```python
from build123d import *

# Parameters (mm, degrees)
SKETCH1_R           = 11.5
SKETCH1_R_2         = 1.4999999999999991
SKETCH1_R_3         = 1.4999999999999987
SKETCH1_R_4         = 1.5000000000000009
SKETCH1_R_5         = 1.5000000000000002
BOSS_EXTRUDE1_DEPTH = 3.5
BOSS_EXTRUDE2_DEPTH = 17.5
CUT_EXTRUDE1_DEPTH  = 73.64483808227534
SKETCH4_R           = 1.3750000000000042
SKETCH4_R_2         = 1.375000000000001
CUT_EXTRUDE2_DEPTH  = 266.22147666332955
FILLET1_R           = 2.5
FILLET2_R           = 1


with BuildPart() as part:
    # Sketch1 → Boss-Extrude1 (new body)
    with BuildSketch(Plane.XY):
        with BuildLine():
            Line((-20.5, -16.000000000000007), (-15.999999999999996, -20.500000000000007))
            Line((-15.999999999999996, -20.500000000000007), (16.000000000000004, -20.5))
            Line((16.000000000000004, -20.5), (20.5, -16))
            Line((20.5, -16), (20.5, 16))
            Line((20.5, 16), (16.000000000000004, 20.5))
            Line((16.000000000000004, 20.5), (-23.500000000000007, 20.5))
            Line((-23.500000000000007, 20.5), (-23.500000000000007, 33))
            Line((-23.500000000000007, 33), (-41.00000000000001, 33))
            Line((-41.00000000000001, 33), (-41.00000000000001, 22.75))
            Line((-41.00000000000001, 22.75), (-35.22649730810378, 12.75))
            Line((-35.22649730810378, 12.75), (-29.500000000000007, 12.750000000000002))
            ThreePointArc((-29.500000000000007, 12.750000000000002), (-23.136038969321078, 10.11396103067893), (-20.500000000000004, 3.750000000000001))
            Line((-20.500000000000004, 3.750000000000001), (-20.5, -16.000000000000007))
        make_face()
        Circle(SKETCH1_R, mode=Mode.SUBTRACT)
        with Locations((-15.500000000000002, 15.5)):
            Circle(SKETCH1_R_2, mode=Mode.SUBTRACT)
        with Locations((15.500000000000002, 15.499999999999998)):
            Circle(SKETCH1_R_3, mode=Mode.SUBTRACT)
        with Locations((15.5, -15.5)):
            Circle(SKETCH1_R_4, mode=Mode.SUBTRACT)
        with Locations((-15.5, -15.5)):
            Circle(SKETCH1_R_5, mode=Mode.SUBTRACT)
        with Locations((-30.00000000000001, 20.746197723675813)):
            Circle(SKETCH1_R_4, mode=Mode.SUBTRACT)
    extrude(amount=BOSS_EXTRUDE1_DEPTH)

    # Sketch2 → Boss-Extrude2 (add)
    with BuildSketch(Plane.ZY.offset(41.00000000000001)):
        Polygon((3.5, 33), (20.15, 33), (20.15, 27.000000000000004), (3.5, 22.75), align=None)
    extrude(amount=-BOSS_EXTRUDE2_DEPTH)

    # Sketch3 → Cut-Extrude1 (cut, through all)
    with BuildSketch(Plane.ZY.offset(41.00000000000001)):
        with BuildLine():
            Line((0, 26.060862236758553), (0, 38.04576260464925))
            Line((0, 38.04576260464925), (20.15, 38.04576260464925))
            Line((20.15, 38.04576260464925), (20.149999999999995, 30.990381056766584))
            ThreePointArc((20.149999999999995, 30.990381056766584), (9.085499481104915, 32.57032381420525), (0, 26.060862236758553))
        make_face()
    extrude(amount=-CUT_EXTRUDE1_DEPTH, mode=Mode.SUBTRACT)

    # Sketch4 → Cut-Extrude2 (cut, through all)
    with BuildSketch(Plane(origin=(-1.4737e-13, -20.499999999999993, -236.3635116976825), x_dir=(1, 2.2e-16, 0), z_dir=(-2.2e-16, 1, 0))):
        with Locations((-35.99999999999985, -249.01351169768247)):
            Circle(SKETCH4_R)
        with Locations((-28.499999999999844, -249.01351169768247)):
            Circle(SKETCH4_R_2)
    extrude(amount=CUT_EXTRUDE2_DEPTH, mode=Mode.SUBTRACT)

    # Fillet1
    # the kernel refuses this fillet: 2.5 mm, written as the material it adds along each edge
    with BuildSketch(Plane(origin=(-41.00000000000001, 22.75, 3.5), x_dir=(0, -1, 0), z_dir=(1, 0, 0))) as fillet1_piece_1_section:
        with BuildLine():
            CenterArc((FILLET1_R * 0.776808330642, -FILLET1_R), FILLET1_R, 90, 75.68071687498136)
            Line((-FILLET1_R * 0.192124217376, -FILLET1_R * 0.752674875131), (0, 0))
            Line((0, 0), (FILLET1_R * 0.776808330642, 0))
        make_face()
    fillet1_piece_1 = extrude(amount=17.5, mode=Mode.PRIVATE)
    fillet1_piece_1 = split(fillet1_piece_1, bisect_by=Plane(origin=(-38.678687412646255, 18.729368658454117, 3.931557915234251), z_dir=(0.8660254037844398, 0.49999999999999795, 0)), keep=Keep.TOP, mode=Mode.PRIVATE)
    fillet1_piece_1 = fillet1_piece_1 - Plane(origin=(-30.00000000000001, 20.746197723675813, 3.931557915234251), x_dir=(1, 0, 0), z_dir=(0, 0, -1)) * Cylinder(1.5000000000000009, 43, mode=Mode.PRIVATE)
    add(fillet1_piece_1)
    # the kernel refuses this fillet: 2.5 mm, written as the material it takes off along each edge
    with BuildSketch(Plane(origin=(-45.855052066513494, 27.000000000000004, 20.15), x_dir=(0, 1, 0), z_dir=(1, 0, 0))) as fillet1_2_piece_1:
        with BuildLine():
            CenterArc((FILLET1_R * 0.776808330642, -FILLET1_R), FILLET1_R, 90, 75.68071687498119)
            Line((-FILLET1_R * 0.192124217376, -FILLET1_R * 0.752674875131), (0, 0))
            Line((0, 0), (FILLET1_R * 0.776808330642, 0))
        make_face()
    extrude(amount=27.21010413302697, mode=Mode.SUBTRACT)

    # Fillet2
    fillet2_edges = [part.edges().sort_by_distance(p)[0] for p in [
        (-41.00000000000001, 24.875, 11.825),
        (-23.500000000000007, 24.875, 11.825),
        (-41.00000000000001, 29.96620094168579, 20.15),
        (-41, 27.408362134202072, 19.624307730627862),
        (-23.500000000000007, 29.96620094168579, 20.15),
        (-23.5, 27.408362134202072, 19.624307730627862),
        (-41, 23.04189744334401, 4.877676890023187),
        (-23.5, 22.341637865797928, 4.025692269372136),
        (-41, 22.749999999999133, 2.2128286226876686),
        (-23.500000000000007, 20.6539895866975, 3.5),
    ]]
    fillet(fillet2_edges, radius=FILLET2_R)


solid = part.part
```
Geometry check sheet. Reference: the model listing, model coordinates, mm. A direction names the side the tool comes from. Give positions to 0.01 mm unless a question says otherwise; leave off trailing zeros. Write each loop counter-clockwise with the first axis right and the second up, starting at its lowest first coordinate (ties: lowest second). Pieces come first, ordered by that corner, then holes.
1) Release check for a two-part mould opening along Y. For faces 1 (the flat face through (-20.5, -6, 2)), 2 (the cylindrical face through (-30.195, 22.233, 1.95)), 3 (the cylindrical face through (-32.36, 22.32, 4.01)), 4 (the cylindrical face through (14, -15.43, 1.73)) record: pulls with the +Y half, pulls with the -Y half, needs draft (parallel to the pull), parting line crosses it, or undercut.
2) Section check A-A, the plane x = 0. Record the boundary of the cut face in (y, z), and give its area (3 significant figures).
3) Gauge pin test, flat ends, axial feed: pin 1 (12 mm diameter, centred on x = 14, y = 25, fed in from +Z); pin 2 (1.8 mm diameter, centred on y = -8, z = 2, fed in from -X); pin 3 (10 mm diameter, centred on x = 3.5, z = 8, fed in from +Y); pin 4 (1 mm diameter, centred on x = -6, y = -8, fed in from -Z). Record the tip position at first contact, or that the pin passes through.
4) Material ranges on L1, parallel to X at y = 29.25, z = 12.65 (3 decimals); L2, parallel to Y at x = -15.5, z = 2.2; L3, parallel to X at y = 28.5, z = 12, recorded low to high.
5) Section check B-B, the plane y = -4.5. Record the boundary of the cut face in (x, z), and give its area (3 significant figures).
6) Section check C-C, the plane x = -36. Record the boundary of the cut face in (y, z) (3 decimals), and give its area (3 significant figures).
7) Access from +Z, -Z, +X, -X, +Y, -Y to the whole of each face (thin tool, end or side, straight path). Record for faces 5 (the flat face through (18.2, -18.3, 1.7)), 6 (the flat face through (-32, 12.75, 2)).
Computed:
1. face 1: needs draft
1. face 2: undercut
1. face 3: pulls with the -Y half
1. face 4: undercut
2. outline: (-20.5, 0) - (-11.5, 0) - (-11.5, 3.5) - (-20.5, 3.5) - close; (11.5, 0) - (20.5, 0) - (20.5, 3.5) - (11.5, 3.5) - close
2. area: 63.0 mm2
3. pin 1: stops at z = 3.5
3. pin 2: stops at x = -20.5
3. pin 3: stops at y = 20.5
3. pin 4: passes through
4. L1: x = -41 to -37.375, -34.625 to -29.875, -27.125 to -23.5
4. L2: y = -20.5 to -17, -14 to 14, 17 to 20.5
4. L3: x = -41 to -37.21, -34.79 to -29.71, -27.29 to -23.5
5. outline: (-20.5, 0) - (-10.58, 0) - (-10.58, 3.5) - (-20.5, 3.5) - close; (10.58, 0) - (20.5, 0) - (20.5, 3.5) - (10.58, 3.5) - close
5. area: 69.4 mm2
6. outline: (14.09, 0) - (26.061, 0) arc R15 ccw to (32.937, 11.275) - (24.735, 11.275) - (23.23, 5.382) arc R2.5 cw to (20.808, 3.5) - (14.09, 3.5) - close; (25.437, 14.025) - (32.937, 14.025) arc R15 ccw to (30.99, 20.15) - (28.942, 20.15) arc R2.5 ccw to (26.52, 18.268) - close
6. area: 149 mm2
7. face 5: +Z, -Z, +X, -Y
7. face 6: +Z, -Z, -X, -Y
